from build123d import *

# Parameters (mm, degrees)
SKETCH_1_R          = 10
EXTRUDE_1_DEPTH     = 10
SKETCH_2_W          = 1.600186535
SKETCH_2_H          = 8.27120278
CUT_EXTRUDE_1_DEPTH = 10
CUT_EXTRUDE_2_DEPTH = 2
CUT_EXTRUDE_3_DEPTH = 2
CUT_EXTRUDE_4_DEPTH = 3.5
CUT_EXTRUDE_5_DEPTH = 8
SKETCH_16_W         = 6
SKETCH_16_H         = 9.252604953
CUT_EXTRUDE_7_DEPTH = 1
SKETCH_17_R         = 3.5
CUT_EXTRUDE_8_DEPTH = 1
SKETCH_18_R         = 3.5
CUT_EXTRUDE_9_DEPTH = 1
SKETCH_19_W         = 3.5
SKETCH_19_H         = 1
EXTRUDE_2_DEPTH     = 4
SKETCH_20_W         = 3.5
SKETCH_20_H         = 1
EXTRUDE_3_DEPTH     = 4
SKETCH_21_W         = 3.540013918
SKETCH_21_H         = 5.43980515
EXTRUDE_4_DEPTH     = 1


with BuildPart() as part:
    # 草圖1 → 填料-伸長1 (new body)
    with BuildSketch(Plane.XY):
        Circle(SKETCH_1_R)
    extrude(amount=EXTRUDE_1_DEPTH)

    # 草圖2 → 除料-伸長1 (cut)
    with BuildSketch(Plane.XY.offset(10)):
        with Locations((-5.134616168, 0.535617876)):
            Rectangle(SKETCH_2_W, SKETCH_2_H)
    extrude(amount=-CUT_EXTRUDE_1_DEPTH, mode=Mode.SUBTRACT)

    # 草圖3 → 除料-伸長2 (cut)
    with BuildSketch(Plane.XY.offset(10)):
        with BuildLine():
            Line((-5.934709435, 4.671219266), (-8.84192912, 4.671219266))
            ThreePointArc((-8.84192912, 4.671219266), (-10.338729016, 0.052381637), (-8.888807861, -4.581385687))
            Line((-8.888807861, -4.581385687), (-5.934709435, -3.599983514))
            Line((-5.934709435, -3.599983514), (-5.934709435, 4.671219266))
        make_face()
    extrude(amount=-CUT_EXTRUDE_2_DEPTH, mode=Mode.SUBTRACT)

    # 草圖4 → 除料-伸長3 (cut)
    with BuildSketch(Plane(origin=(0, 0, 0), x_dir=(-1, 0, 0), z_dir=(0, 0, -1))):
        with BuildLine():
            Line((5.934709435, 4.671219266), (8.84192912, 4.671219266))
            ThreePointArc((8.84192912, 4.671219266), (10.34374886, 0.021931836), (8.86165829, -4.633682375))
            Line((8.86165829, -4.633682375), (5.934709435, -4.633682375))
            Line((5.934709435, -4.633682375), (5.934709435, 4.671219266))
        make_face()
    extrude(amount=-CUT_EXTRUDE_3_DEPTH, mode=Mode.SUBTRACT)

    # 草圖7 → 除料-伸長4 (cut)
    with BuildSketch(Plane.ZY.offset(13.3345229)):
        Polygon((2, 4.671219266), (8, 4.671219266), (8, -4.581385687), (2, -4.633682375), align=None)
    extrude(amount=-CUT_EXTRUDE_4_DEPTH, mode=Mode.SUBTRACT)

    # 草圖9 → 除料-伸長5 (cut)
    with BuildSketch(Plane.XY.offset(8)):
        Polygon((-5.934709435, 4.614635236), (-5.934709435, -3.599983514), (-6.581816343, -3.814963529), (-6.581816343, 4.614635236), align=None)
    extrude(amount=-CUT_EXTRUDE_5_DEPTH, mode=Mode.SUBTRACT)

    # 草圖16 → 除料-伸長7 (cut)
    with BuildSketch(Plane.ZY.offset(9.8345229)):
        with Locations((5, 0.04491679)):
            Rectangle(SKETCH_16_W, SKETCH_16_H)
    extrude(amount=-CUT_EXTRUDE_7_DEPTH, mode=Mode.SUBTRACT)

    # 草圖17 → 除料-伸長8 (cut)
    with BuildSketch(Plane(origin=(0, 0, 0), x_dir=(-1, 0, 0), z_dir=(0, 0, -1))):
        with Locations((-3.576623966, 1.840103877)):
            Circle(SKETCH_17_R)
    extrude(amount=-CUT_EXTRUDE_8_DEPTH, mode=Mode.SUBTRACT)

    # 草圖18 → 除料-伸長9 (cut)
    with BuildSketch(Plane.XY.offset(10)):
        with Locations((4.177553206, 2.507636002)):
            Circle(SKETCH_18_R)
    extrude(amount=-CUT_EXTRUDE_9_DEPTH, mode=Mode.SUBTRACT)

    # 草圖19 → 填料-伸長2 (add)
    with BuildSketch(Plane(origin=(9.418183657, 0, 0), x_dir=(0, 0, -1), z_dir=(1, 0, 0))):
        with Locations((-5.219032707, 3.16388309)):
            Rectangle(SKETCH_19_W, SKETCH_19_H)
    extrude(amount=EXTRUDE_2_DEPTH)

    # 草圖20 → 填料-伸長3 (add)
    with BuildSketch(Plane(origin=(9.418183657, 0, 0), x_dir=(0, 0, -1), z_dir=(1, 0, 0))):
        with Locations((-5.179018789, -1.27592206)):
            Rectangle(SKETCH_20_W, SKETCH_20_H)
    extrude(amount=EXTRUDE_3_DEPTH)

    # 草圖21 → 填料-伸長4 (add)
    with BuildSketch(Plane(origin=(13.418183657, 0, 0), x_dir=(0, 0, -1), z_dir=(1, 0, 0))):
        with Locations((-5.199025748, 0.943980515)):
            Rectangle(SKETCH_21_W, SKETCH_21_H)
    extrude(amount=EXTRUDE_4_DEPTH)


solid = part.part
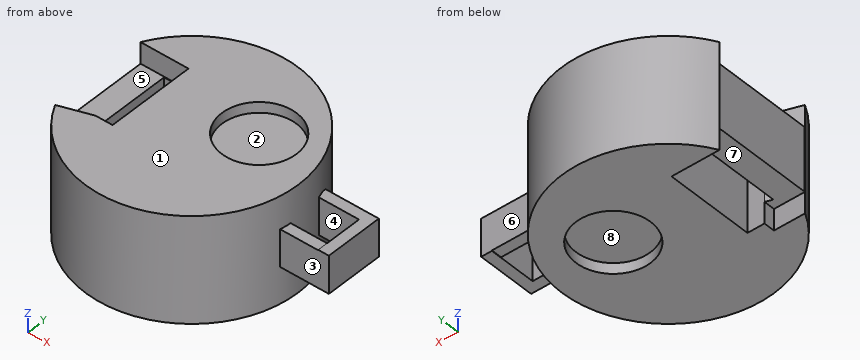
Could you check a few things on this model? Use its own coordinates, in mm. Face numbers are marked on the shaded views. A direction names the side the tool comes from. Give positions to 0.01 mm unless a question says otherwise; leave off trailing zeros. Order: outer loops, then holes, each group sorted by start corner. A loop starts at its lowest first (then second) coordinate and runs counter-clockwise, first axis right, second up. Notation, with made-up numbers: M 8.25,5 L 36.25,5 A15 ccw 36.25,13 Z; hole C 78.5,78.5 d10. An arc over 180 degrees is marked long. One line per question, with ' | ' between items.
1. I want a section at D-D (x = 3.75). List the corners of the cut face in (y, z) for me, and give its area (3 significant figures).
Results:
outline: M -9.27,0 L -1.66,0 L -1.66,1 L 5.34,1 L 5.34,0 L 9.27,0 L 9.27,10 L 5.98,10 L 5.98,9 L -0.97,9 L -0.97,10 L -9.27,10 Z | area: 171 mm²
2. I want a section at B-B (x = -5). List the corners of the cut face in (y, z) for me.
Results:
outline: M -8.66,0 L -3.6,0 L -3.6,10 L -8.66,10 Z; M 4.67,0 L 8.66,0 L 8.66,10 L 4.67,10 Z
3. I'm going to push flat-ended pins straight in: pin 1 (6 mm diameter, centred on y = 6, z = 6, fed in from -X); pin 2 (1.1 mm diameter, centred on y = -4.5, z = 1, fed in from -X); pin 3 (2 mm diameter, centred on x = -1.5, z = 6, fed in from +Y). Where does each tip first touch, or does it pass through?
Results:
pin 1: x = -8.84 | pin 2: x = -8.86 | pin 3: y = 9.99
4. We'd pull the mould along Y, two halves only. Please class the marked faces 1, 2 and 3: +Y half, -Y half, draft (parallel to the pull), parting line (faces both ways), or undercut.
Results:
face 1: draft | face 2: undercut | face 3: -Y half
5. I want a section at C-C (y = -2.5). List the corners of the cut face in (x, z) for me, and give its area (3 significant figures).
Results:
outline: M -8.83,2 L -6.58,2 L -6.58,8 L -8.83,8 Z; M -4.33,0 L 9.68,0 L 9.68,10 L -4.33,10 Z | area: 154 mm²
6. If I drill on line 1 (X direction, y = 1.75, z = 0.5); line 2 (X direction, y = 2.5, z = 6); line 3 (X direction, y = -0.5, z = 5.75), over which ranges is the centre line in solid material (lowest first)?
Results:
line 1: -4.33 to 0.08, 7.08 to 9.85 | line 2: -8.83 to -6.58, -4.33 to 9.68, 13.42 to 14.42 | line 3: -8.83 to -6.58, -4.33 to 9.99, 13.42 to 14.42
7. For the marked faces 4, 5, 6, 7 and 8, which set-ups out of +Z, -Z, +X, -X, +Y, -Y let a thin tool reach every point of the face, with its end or its side?
Results:
face 4: +Z, -Z | face 5: +Z, -X | face 6: +Z, -Z, +X, +Y | face 7: -Z, -X | face 8: -Z
8. I want a section at A-A (y = -0.5). List the corners of the cut face in (x, z) for me.
Results:
outline: M -8.83,2 L -6.58,2 L -6.58,8 L -8.83,8 Z; M -4.33,0 L 0.97,0 L 0.97,1 L 6.18,1 L 6.18,0 L 9.99,0 L 9.99,10 L 5.97,10 L 5.97,9 L 2.39,9 L 2.39,10 L -4.33,10 Z; M 13.42,3.43 L 14.42,3.43 L 14.42,6.97 L 13.42,6.97 Z
